```python
from build123d import *

# Parameters (mm, degrees)
EXTRUDE_1_DEPTH = 4
SKETCH_2_R      = 3
SKETCH_2_R_2    = 2.1
EXTRUDE_2_DEPTH = 3.2
FILLET_1_R      = 0.3


with BuildPart() as part:
    # Эскиз1 → Бобышка-Вытянуть1 (new body)
    with BuildSketch(Plane(origin=(0, 0, 0), x_dir=(1, 0, 0), z_dir=(0, 1, 0))):
        with BuildLine():
            Line((6, 6), (-6, 6))
            ThreePointArc((-6, 6), (-12, 0), (-6, -6))
            Line((-6, -6), (6, -6))
            ThreePointArc((6, -6), (12, 0), (6, 6))
        make_face()
    extrude(amount=EXTRUDE_1_DEPTH)

    # Эскиз2 → Бобышка-Вытянуть2 (add)
    # profile 1 of 2: a face of its own
    with BuildSketch(Plane(origin=(0, 4, 0), x_dir=(1, 0, 0), z_dir=(0, 1, 0))):
        with Locations(Location((6.5, 0, 0), (0, 0, 90))):
            Circle(SKETCH_2_R)
        with Locations(Location((6.5, 0, 0), (0, 0, 270))):
            Circle(SKETCH_2_R_2, mode=Mode.SUBTRACT)
    # profile 2 of 2: a face of its own
    with BuildSketch(Plane(origin=(0, 4, 0), x_dir=(1, 0, 0), z_dir=(0, 1, 0))):
        Polygon((-1.881197846, 0), (-4.190598923, 4), (-8.809401077, 4), (-11.118802154, 0), (-8.809401077, -4), (-4.190598923, -4), align=None)
        Polygon((-3.4977786, 0), (-4.9988893, 2.6), (-8.0011107, 2.6), (-9.5022214, 0), (-8.0011107, -2.6), (-4.9988893, -2.6), align=None, mode=Mode.SUBTRACT)
    extrude(amount=EXTRUDE_2_DEPTH)

    # Скругление1
    fillet_1_edges = [part.edges().sort_by_distance(p)[0] for p in [
        (6.5, 7.2, 3),
        (6.5, 7.2, -2.1),
        (-3.035898385, 7.2, 2),
        (-3.035898385, 7.2, -2),
        (-6.5, 7.2, -4),
        (-9.964101615, 7.2, -2),
        (-9.964101615, 7.2, 2),
        (-6.5, 7.2, 4),
        (-4.24833395, 7.2, 1.3),
        (-4.24833395, 7.2, -1.3),
        (-6.5, 7.2, -2.6),
        (-8.75166605, 7.2, -1.3),
        (-8.75166605, 7.2, 1.3),
        (-6.5, 7.2, 2.6),
    ]]
    fillet(fillet_1_edges, radius=FILLET_1_R)


solid = part.part
```
CAD build for the part. Positions are in the model's coordinates, mm. A direction names the side the tool comes from. Round coordinates to 2 decimals unless told otherwise and drop trailing zeros. Order: outer loops, then holes, each group sorted by start corner. A loop starts at its lowest first (then second) coordinate and runs counter-clockwise, first axis right, second up. Notation, with made-up numbers: (88, 23) - (119, 23) arc R26 ccw to (119, 58) - close; hole circle Ø8 at (-5.75, 42). An arc over 180 degrees is marked (long way). Answer as CSV lines item,"result". Start each with the question number.
1. Saw through at B-B, the plane x = 6.5. Write the cut outline in (y, z).
2. Pull direction X, two halves, no side cores. Call faces 1 (the face through (-9.87, 7.11, 1.99)), 2 (the face through (6, 4, 0)), 3 (the face through (0, 2, -6)): +X half, -X half, draft (parallel to the pull), parting line (faces both ways), or undercut.
3. Saw through at C-C, the plane z = 5.5. Write the cut outline in (x, y), and give its area (3 significant figures).
4. Saw through at D-D, the plane y = 1.5. Write the cut outline in (x, z).
5. Drill centre lines: L1, parallel to X at y = 5.25, z = -1.25; L2, parallel to X at y = 5, z = 2.5; L3, parallel to Y at x = -8, z = -0.25. Where is each one in solid material? Low to high. Write a range as [from, to].
6. Saw through at A-A, the plane y = 5.75. Write the cut outline in (x, z).
7. Tool access for faces 4 (the face through (-9.948, 5.43, -2.028)), 5 (the face through (-6, 5, -4)), 6 (the face through (-6, 5, -2.6)), 7 (the face through (-7, 5, 4)), 8 (the face through (-3.094, 7.11, 1.929)): list every direction of +Z, -Z, +X, -X, +Y, -Y with a clear straight run to the whole face (end or side of a thin tool).
8. Pin check, flat tips, straight feed: pin 1 (3 mm diameter, centred on x = -2, y = 6, fed in from +Z); pin 2 (1.5 mm diameter, centred on y = 4, z = -1.5, fed in from +X); pin 3 (3 mm diameter, centred on x = -7.5, y = 5, fed in from -Z). Stop position of each tip, or through.
Model answer:
1,outline,"(0, -5.98) - (4, -5.98) - (4, -3) - (6.9, -3) arc R0.3 ccw to (7.2, -2.7) - (7.2, -2.4) arc R0.3 ccw to (6.9, -2.1) - (4, -2.1) - (4, 2.1) - (6.9, 2.1) arc R0.3 ccw to (7.2, 2.4) - (7.2, 2.7) arc R0.3 ccw to (6.9, 3) - (4, 3) - (4, 5.98) - (0, 5.98) - close"
2,face 1,"-X half"
2,face 2,"undercut"
2,face 3,"draft"
3,outline,"(-8.4, 0) - (8.4, 0) - (8.4, 4) - (-8.4, 4) - close"
3,area,"67.2 mm²"
4,outline,"(-6, -6) - (6, -6) arc R6 ccw to (6, 6) - (-6, 6) arc R6 ccw to start"
5,L1,"x = [-10.4, -8.78], [-4.22, -2.6], [3.77, 4.81], [8.19, 9.23]"
5,L2,"x = [-9.68, -8.06], [-4.94, -3.32], [4.84, 8.16]"
5,L3,"y = [0, 4]"
6,outline,"(-11.12, 0) - (-8.81, -4) - (-4.19, -4) - (-1.88, 0) - (-4.19, 4) - (-8.81, 4) - close; circle Ø6 at (6.5, 0); hole (-9.5, 0) - (-8, -2.6) - (-5, -2.6) - (-3.5, 0) - (-5, 2.6) - (-8, 2.6) - close; hole circle Ø4.2 at (6.5, 0)"
7,face 4,"-Z, -X, +Y"
7,face 5,"-Z, +X, -X, +Y"
7,face 6,"+Y"
7,face 7,"+Z, +X, -X, +Y"
7,face 8,"+Z, +Y"
8,pin 1,"stops at z = 2.8"
8,pin 2,"stops at x = 11.95"
8,pin 3,"stops at z = -5.99"
